from build123d import *

# Parameters (mm, degrees)
BOSS_EXTRUDE2_DEPTH = 75
SKETCH2_R           = 4
CUT_EXTRUDE1_DEPTH  = 60
BOSS_EXTRUDE3_DEPTH = 1
SKETCH4_W           = 25
SKETCH4_H           = 20
BOSS_EXTRUDE4_DEPTH = 5
SKETCH5_R           = 9.5
CUT_EXTRUDE5_DEPTH  = 0.3
SKETCH9_R           = 8.5
CUT_EXTRUDE6_DEPTH  = 0.3
SKETCH10_R          = 7.5
CUT_EXTRUDE7_DEPTH  = 0.3
SKETCH11_R          = 6.5
CUT_EXTRUDE8_DEPTH  = 0.3
FILLET1_R           = 2


with BuildPart() as part:
    # Sketch1 → Boss-Extrude2 (new body)
    with BuildSketch(Plane.XY):
        with BuildLine():
            Line((-15.355814747, 10), (14.644185253, 10))
            Line((14.644185253, 10), (14.644185253, 5))
            ThreePointArc((14.644185253, 5), (9.476114191, 3.167336025), (5, 0))
            ThreePointArc((5, 0), (0, -5), (-5, 0))
            ThreePointArc((-5, 0), (-9.810792775, 3.260354155), (-15.355814747, 5))
            Line((-15.355814747, 5), (-15.355814747, 10))
        make_face()
    extrude(amount=-BOSS_EXTRUDE2_DEPTH)

    # Sketch2 → Cut-Extrude1 (cut)
    with BuildSketch(Plane(origin=(0, 0, -75), x_dir=(-1, 0, 0), z_dir=(0, 0, -1))):
        Circle(SKETCH2_R)
    extrude(amount=-CUT_EXTRUDE1_DEPTH, mode=Mode.SUBTRACT)

    # Sketch3 → Boss-Extrude3 (add)
    with BuildSketch(Plane(origin=(0, 10, 0), x_dir=(1, 0, 0), z_dir=(0, 1, 0))):
        with BuildLine():
            Line((-10.355814747, 41), (-10.355814747, 63))
            ThreePointArc((-10.355814747, 63), (-0.355814747, 73), (9.644185253, 63))
            Line((9.644185253, 63), (9.644185253, 41))
            ThreePointArc((9.644185253, 41), (-0.355814747, 31), (-10.355814747, 41))
        make_face()
    extrude(amount=BOSS_EXTRUDE3_DEPTH)

    # Sketch4 → Boss-Extrude4 (add)
    with BuildSketch(Plane(origin=(0, 10, 0), x_dir=(1, 0, 0), z_dir=(0, 1, 0))):
        with Locations((-0.28655183, 14)):
            Rectangle(SKETCH4_W, SKETCH4_H)
    extrude(amount=BOSS_EXTRUDE4_DEPTH)

    # Sketch5 → Cut-Extrude5 (cut)
    with BuildSketch(Plane(origin=(0, 15, 0), x_dir=(1, 0, 0), z_dir=(0, 1, 0))):
        with Locations(Location((0, 14, 0), (0, 0, 270))):
            Circle(SKETCH5_R)
    extrude(amount=-CUT_EXTRUDE5_DEPTH, mode=Mode.SUBTRACT)

    # Sketch9 → Cut-Extrude6 (cut)
    with BuildSketch(Plane(origin=(0, 14.7, 0), x_dir=(1, 0, 0), z_dir=(0, 1, 0))):
        with Locations(Location((0, 14, 0), (0, 0, 270))):
            Circle(SKETCH9_R)
    extrude(amount=-CUT_EXTRUDE6_DEPTH, mode=Mode.SUBTRACT)

    # Sketch10 → Cut-Extrude7 (cut)
    with BuildSketch(Plane(origin=(0, 14.4, 0), x_dir=(1, 0, 0), z_dir=(0, 1, 0))):
        with Locations(Location((0, 14, 0), (0, 0, 270))):
            Circle(SKETCH10_R)
    extrude(amount=-CUT_EXTRUDE7_DEPTH, mode=Mode.SUBTRACT)

    # Sketch11 → Cut-Extrude8 (cut)
    with BuildSketch(Plane(origin=(0, 14.1, 0), x_dir=(1, 0, 0), z_dir=(0, 1, 0))):
        with Locations(Location((0, 14, 0), (0, 0, 270))):
            Circle(SKETCH11_R)
    extrude(amount=-CUT_EXTRUDE8_DEPTH, mode=Mode.SUBTRACT)

    # Sketch12 → Revolve2 (revolve)
    with BuildSketch(Plane(origin=(0, 0, 0), x_dir=(0, 0, -1), z_dir=(1, 0, 0)), mode=Mode.PRIVATE) as revolve2_sk:
        with BuildLine():
            Line((14, 15), (14, 13.677907374))
            Line((14, 13.677907374), (11.5, 13.677907374))
            ThreePointArc((11.5, 13.677907374), (11.70459363, 17.043778802), (10.964658523, 20.333679266))
            Line((10.964658523, 20.333679266), (11.494340347, 23.356462384))
            ThreePointArc((11.494340347, 23.356462384), (12.09773994, 25.084923792), (13, 26.677907374))
            Line((13, 26.677907374), (14, 26.677907374))
            Line((14, 26.677907374), (14, 15))
        make_face()
    revolve(revolve2_sk.sketch.rotate(Axis((0, 13.677907374, -14), (0, 1, 0)), 180), axis=Axis((0, 13.677907374, -14), (0, 1, 0)))

    # Sketch13 → Revolve3 (revolve)
    with BuildSketch(Plane(origin=(0, 0, 0), x_dir=(0, 0, -1), z_dir=(1, 0, 0))):
        with BuildLine():
            Line((14, 23.403548627), (14, 28.403548627))
            ThreePointArc((14, 28.403548627), (17.081597334, 25.903548627), (14, 23.403548627))
        make_face()
    revolve(axis=Axis((0, 23.403548627, -14), (0, 1, 0)))

    # Fillet1
    fillet1_edges = [part.edges().sort_by_distance(p)[0] for p in [
        (-15.355814747, 10, -37.5),
        (14.644185253, 10, -37.5),
        (-0.355814747, 10, 0),
        (-0.355814747, 10, -75),
    ]]
    fillet(fillet1_edges, radius=FILLET1_R - 0.0001)  # a hair under: the kernel refuses the full size


solid = part.part
Here's how the part is built. I have some questions about the finished solid (model axes, mm). A direction names the side the tool comes from. Coordinates: 2 decimals unless noted, no trailing zeros. Order: outer loops, then holes, each group sorted by start corner. A loop starts at its lowest first (then second) coordinate and runs counter-clockwise, first axis right, second up. Notation, with made-up numbers: M 63.25,-9 L 116.25,-9 A10 cw 116.25,7 Z; hole C -6,-14.5 d4. An arc over 180 degrees is marked long. Answer as CSV lines item,"result". Start each with the question number.
1. On a 3-axis mill with a long thin cutter (end or side, diameter ignored), from which of +Z, -Z, +X, -X, +Y, -Y can I reach the whole of each face in a straight line? I mean faces 1 (the flat face through (0, 12, -24)), 2 (the flat face through (0, 12, -4)), 3 (the cylindrical face through (0.867, -3.905, -45.42)), 4 (the conical face through (1.65, 22.2, -11.85)). Say none if no direction works.
2. We'd pull the mould along Z, two halves only. Please class faces 5 (the flat face through (0, 3, 0)), 6 (the flat face through (-9, 15, -19)), 7 (the flat face through (3, 14.1, -20)): released by +Z, released by -Z, zero draft, split by the parting line, or undercut.
3. For pin 1 (1.5 mm diameter, centred on x = -2, z = -57.5, fed in from +Y); pin 2 (1.5 mm diameter, centred on x = -7, y = 2, fed in from +Z); pin 3 (4 mm diameter, centred on y = 20, z = -9.5, fed in from -X); pin 4 (1.5 mm diameter, centred on y = 11.5, z = -17.5, fed in from -X), each with a flat end and sliding along its axis, tell me the tip position at first contact or that it passes through.
4. I need wall thicknesses on line 1 (Y direction, x = 0, z = -47); line 2 (X direction, y = 14.95, z = -14); line 3 (Y direction, x = -2.5, z = -39.5). Which ranges of each line are inside material? Lowest first, please. Write a range as [from, to].
5. I want a section at B-B, the plane y = 2. Write out the boundary of the cut face in (x, z).
6. I want a section at A-A, the plane z = -45.5. Write out the boundary of the cut face in (x, y), and give its area (3 significant figures).
7. I want a section at C-C, the plane z = -29.5. Write out the boundary of the cut face in (x, y).
8. I want a section at D-D, the plane z = -69.5. Write out the boundary of the cut face in (x, y).
Recorded:
1,face 1,"+X, -X, +Y"
1,face 2,"+Z, +X, -X, +Y"
1,face 3,"-Z"
1,face 4,"none"
2,face 5,"released by +Z"
2,face 6,"zero draft"
2,face 7,"undercut"
3,pin 1,"stops at y = 11"
3,pin 2,"stops at z = 0"
3,pin 3,"stops at x = -1.68"
3,pin 4,"stops at x = -12.79"
4,line 1,"y = [-5, -4], [4, 11]"
4,line 2,"x = [-12.79, -9.5], [-2.31, 2.31], [9.5, 12.21]"
4,line 3,"y = [-4.33, -3.12], [3.12, 11]"
5,outline,"M -7.58,-75 L -3.46,-75 L -3.46,-15 L 3.46,-15 L 3.46,-75 L 7.51,-75 L 7.51,0 L -7.58,0 Z"
6,outline,"M -15.36,5 A20 cw -5,0 A5 ccw 5,0 A20 cw 14.64,5 L 14.64,8 A2 ccw 12.64,10 L 9.64,10 L 9.64,11 L -10.36,11 L -10.36,10 L -13.36,10 A2 ccw -15.36,8 Z; hole C 0,0 d8"
6,area,"245 mm2"
7,outline,"M -15.36,5 A20 cw -5,0 A5 ccw 5,0 A20 cw 14.64,5 L 14.64,8 A2 ccw 12.64,10 L -13.36,10 A2 ccw -15.36,8 Z; hole C 0,0 d8"
8,outline,"M -15.36,5 A20 cw -5,0 A5 ccw 5,0 A20 cw 14.64,5 L 14.64,8 A2 ccw 12.64,10 L 7.24,10 L 7.24,11 L -7.96,11 L -7.96,10 L -13.36,10 A2 ccw -15.36,8 Z; hole C 0,0 d8"
